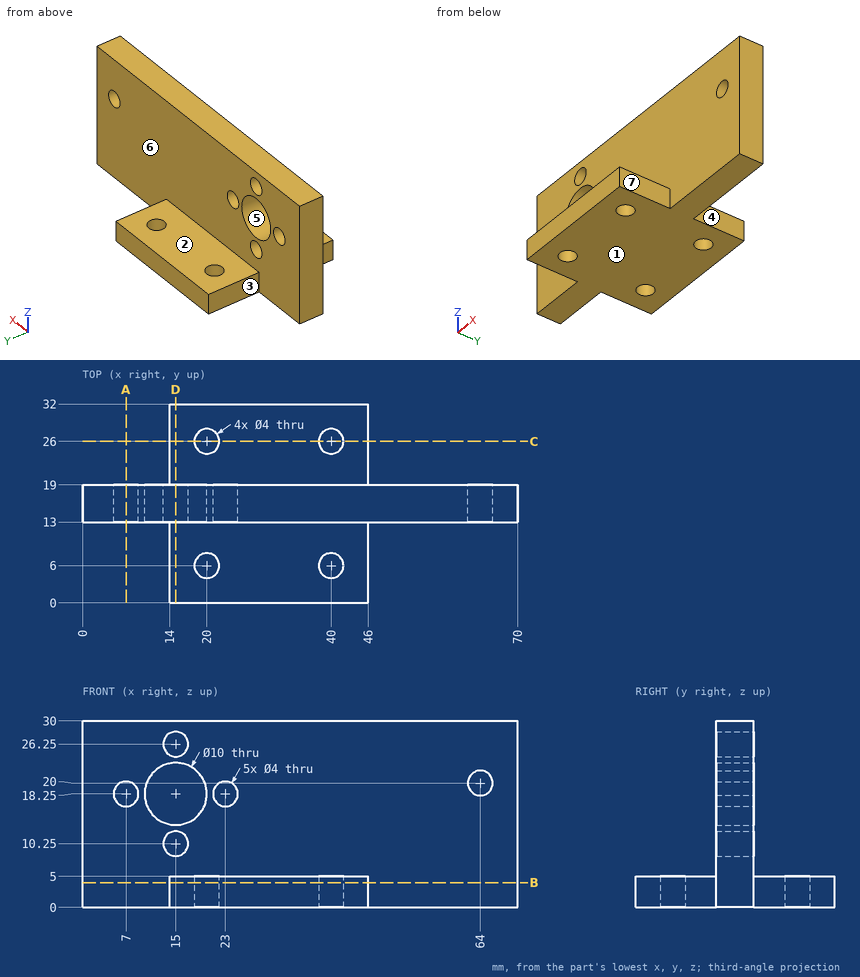
Check sheet for the drawn part. Datum: minimum x, y, z corner. Units: mm. A direction names the side the tool comes from. Give positions to 0.01 mm unless a question says otherwise; leave off trailing zeros. Loops run counter-clockwise (first coordinate to the right, second up) from the corner with the lowest first, then second, coordinate; pieces in that order, holes last. Notation, with made-up numbers: M -28.5,-21 L -10.5,-21 A16 ccw -10.5,9 Z; hole C 50.25,3.5 d4. An arc over 180 degrees is marked long. Return JSON: item names as keys, results as strings.
1) Gauge pin test, flat ends, axial feed: P1, Ø2.5, axis at y = 4, z = 2, coming from the +X side; P2, Ø4, axis at x = 27.5, y = 7, coming from the +Z side; P3, Ø5, axis at x = 15, z = 10.25, coming from the +Y side. Record the tip position at first contact, or that the pin passes through.
Findings:
{"P1": "stops at x = 46", "P2": "stops at z = 5", "P3": "stops at y = 19"}
2) Section check D-D, the plane x = 15. Enter the section's corners in (y, z), and give its area (3 significant figures).
Findings:
{"outline": "M 0,0 L 32,0 L 32,5 L 19,5 L 19,8.25 L 13,8.25 L 13,5 L 0,5 Z; M 13,12.25 L 19,12.25 L 19,13.25 L 13,13.25 Z; M 13,23.25 L 19,23.25 L 19,24.25 L 13,24.25 Z; M 13,28.25 L 19,28.25 L 19,30 L 13,30 Z", "area": "202 mm2"}
3) Section check A-A, the plane x = 7. Enter the section's corners in (y, z), and give its area (3 significant figures).
Findings:
{"outline": "M 13,0 L 19,0 L 19,16.25 L 13,16.25 Z; M 13,20.25 L 19,20.25 L 19,30 L 13,30 Z", "area": "156 mm2"}
4) Tool access check on the marked faces 1, 2, 3 and 4. Record the directions out of +Z, -Z, +X, -X, +Y, -Y that give a thin tool (end or side, any length) a straight path to the whole face; none if there is none.
Findings:
{"face 1": "-Z, +X, -X, +Y, -Y", "face 2": "+Z, +X, -X, +Y", "face 3": "+Z, -Z, -X, +Y", "face 4": "+Z, -Z, +X, +Y"}
5) Section check B-B, the plane z = 4. Enter the section's corners in (x, y), and give its area (3 significant figures).
Findings:
{"outline": "M 0,13 L 14,13 L 14,0 L 46,0 L 46,13 L 70,13 L 70,19 L 46,19 L 46,32 L 14,32 L 14,19 L 0,19 Z; hole C 20,6 d4; hole C 20,26 d4; hole C 40,6 d4; hole C 40,26 d4", "area": "1,200 mm2"}
6) Mould release check, pull along X, two halves, no side actions. Record for the marked faces 5, 6 and 7: released by +X, released by -X, zero draft, split by the parting line, or undercut.
Findings:
{"face 5": "undercut", "face 6": "zero draft", "face 7": "released by +X"}
7) Material ranges on L1, parallel to Y at x = 20, z = 1.45; L2, parallel to Z at x = 64, y = 14; L3, parallel to Z at x = 7, y = 15.5, recorded low to high. Write a range as [from, to].
Findings:
{"L1": "y = [0, 4], [8, 24], [28, 32]", "L2": "z = [0, 18], [22, 30]", "L3": "z = [0, 16.25], [20.25, 30]"}
8) Section check C-C, the plane y = 26. Enter the section's corners in (x, z).
Findings:
{"outline": "M 14,0 L 18,0 L 18,5 L 14,5 Z; M 22,0 L 38,0 L 38,5 L 22,5 Z; M 42,0 L 46,0 L 46,5 L 42,5 Z"}
